Autodesk Fusion 360 part; units mm, degrees
sketch "Esquisse4" plane through (0, 0, 0) normal (0, 1, 0) x (1, 0, 0)
  line L0 (-8.2212, 10.9612) -> (-33.2212, 10.9612)
  line L1 (-33.2212, 10.9612) -> (-33.2212, -14.0388)
  line L2 (-33.2212, -14.0388) -> (-8.2212, -14.0388)
  line L3 (-8.2212, -14.0388) -> (-8.2212, 10.9612)
  dimension "d13" = 25
  dimension "d14" = 25
extrude "Extrusion4" add sketch "Esquisse4" along normal blind 25
sketch "Esquisse5" plane through (0, 25, 0) normal (0, 1, 0) x (-1, 0, 0)
  line L0 (8.2212, 14.0388) -> (8.2212, -10.9612)
  line L1 (8.2212, -10.9612) -> (33.2212, -10.9612)
  line L2 (33.2212, -10.9612) -> (33.2212, 14.0388)
  line L3 (33.2212, 14.0388) -> (8.2212, 14.0388)
  circle A0 centre (20.7212, 1.5388) radius 1.5
  line L4 (33.2212, -10.9612) -> (8.2212, 14.0388) construction
  dimension "d19" = 3
extrude "Extrusion5" cut sketch "Esquisse5" against normal blind 0.5 contours A0
sketch "Esquisse7" plane through (0, 0, 14.0388) normal (0, 0, 1) x (1, 0, 0)
  line L0 (-33.2212, 0) -> (-8.2212, 0)
  line L1 (-8.2212, 0) -> (-8.2212, 25)
  line L2 (-8.2212, 25) -> (-33.2212, 25)
  line L3 (-33.2212, 25) -> (-33.2212, 0)
  line L4 (-33.2212, 25) -> (-8.2212, 0) construction
  line L5 (-33.2212, 0) -> (-8.2212, 25) construction
  circle A0 centre (-20.7212, 12.5) radius 1.5
  circle A1 centre (-27.7923, 19.5711) radius 1.5
  circle A2 centre (-13.6501, 5.4289) radius 1.5
  dimension "d20" = 3
  dimension "d21" = 10
extrude "Extrusion6" cut sketch "Esquisse7" against normal blind 0.5 contours A0 | A1 | A2
sketch "Esquisse8" plane through (-8.2212, 0, 0) normal (1, 0, 0) x (0, 0, -1)
  line L0 (-14.0388, 0) -> (10.9612, 0)
  line L1 (10.9612, 0) -> (10.9612, 25)
  line L2 (10.9612, 25) -> (-14.0388, 25)
  line L3 (-14.0388, 25) -> (-14.0388, 0)
  line L4 (-14.0388, 25) -> (10.9612, 0) construction
  circle A0 centre (-1.5388, 12.5) radius 1.5
  line L5 (-14.0388, 0) -> (10.9612, 25) construction
  circle A1 centre (-8.6098, 19.5711) radius 1.5
  circle A2 centre (-8.6098, 5.4289) radius 1.5
  circle A3 centre (5.5323, 5.4289) radius 1.5
  circle A4 centre (5.5323, 19.5711) radius 1.5
  dimension "d24" = 3
  dimension "d25" = 3
  dimension "d27" = 360
  dimension "d28" = 10
extrude "Extrusion7" cut sketch "Esquisse8" against normal blind 0.5 contours A0 | A1 | A2 | A3 | A4
fillet "Congé2" radius 2.5 12 edges at (-20.7212, 25, 14.0388) (-8.2212, 25, 1.5388) (-8.2212, 12.5, 14.0388) (-33.2212, 12.5, 14.0388) (-33.2212, 25, 1.5388) (-33.2212, 12.5, -10.9612) (-33.2212, 0, 1.5388) (-20.7212, 25, -10.9612) (-8.2212, 12.5, -10.9612) (-20.7212, 0, -10.9612) (-8.2212, 0, 1.5388) (-20.7212, 0, 14.0388)
sketch "Esquisse9" plane through (0, 0, 0) normal (1, 0, 0) x (0, 0, -1)
  circle A0 centre (-30.7056, 27.1014) radius 10
  dimension "d33" = 20
equation "d14 = d13"
equation "d15 = d13"
Design review of the part built by this model. Coordinates are the model's own, in mm. A direction names the side the tool comes from. Coordinates: 2 decimals unless noted, no trailing zeros. Loops run counter-clockwise (first coordinate to the right, second up) from the corner with the lowest first, then second, coordinate; pieces in that order, holes last.
Item 1: For faces 1 (the cylindrical face through (-8.973, 12.64, 13.326)), 2 (the flat face through (-28, 20, 13.539)), 3 (the flat face through (-21, 24.5, 2)), 4 (the flat face through (-8.721, 13, 2)), list the 3-axis set-ups (+Z, -Z, +X, -X, +Y, -Y) from which the entire face can be reached by the end or side of a thin tool; tool diameter is ignored.
Completed:
face 1: +Z, +X, +Y, -Y
face 2: +Z
face 3: +Y
face 4: +X
Item 2: Wall thickness on L1, parallel to X at y = 6, z = 7.5; L2, parallel to X at y = 5.5, z = 12.25; L3, parallel to Z at x = -21.5, y = 23.5: over which ranges is each line inside the solid? List them lowest first.
Completed:
L1: x = -33.22 to -8.72
L2: x = -33.12 to -8.32
L3: z = -10.75 to 13.83
Item 3: Draft analysis for pull direction Z (two halves, no side actions). For faces 5 (the cylindrical face through (-8.5, 18.1, 8.9)), 6 (the cylindrical face through (-22.22, 12.57, 13.79)), 7 (the cylindrical face through (-20.581, 24.287, 13.287)), 8 (the cylindrical face through (-20.861, 24.287, -10.209)), state which applies: pulls with the +Z half, pulls with the -Z half, needs draft (parallel to the pull), parting line crosses it, or undercut.
Completed:
face 5: undercut
face 6: needs draft
face 7: pulls with the +Z half
face 8: pulls with the -Z half
Item 4: Clearance check with flat-ended pins moving along their axes: pin 1 (0.9 mm diameter, centred on y = 5.5, z = 8.5, fed in from +X); pin 2 (1.5 mm diameter, centred on x = -21, y = 12.5, fed in from +Z); pin 3 (3 mm diameter, centred on x = -14.5, z = -4, fed in from -Y). State where each tip first meets the part, or that it passes through.
Completed:
pin 1: stops at x = -8.72
pin 2: stops at z = 13.54
pin 3: stops at y = 0
Item 5: Add section A-A (x = -10). Write out the cut boundary in (y, z), and give its area (3 significant figures).
Completed:
outline: (0.11, -8.46) arc R2.39 ccw to (2.5, -10.85) - (22.5, -10.85) arc R2.39 ccw to (24.89, -8.46) - (24.89, 11.54) arc R2.39 ccw to (22.5, 13.93) - (2.5, 13.93) arc R2.39 ccw to (0.11, 11.54) - close
area: 609 mm2
